Read the model definition and answer for the solid it produces. Units are mm, in the model's axes. Face numbers are marked on the shaded views. A direction names the side the tool comes from. Coordinates: 2 decimals unless noted, no trailing zeros. Loops run counter-clockwise (first coordinate to the right, second up) from the corner with the lowest first, then second, coordinate; pieces in that order, holes last. Notation, with made-up numbers: (72.5, 6.25) -> (111.5, 6.25) arc R11 cw to (111.5, 15.25) -> close; hole circle Ø6 at (-30.5, 60.25). An arc over 180 degrees is marked (long way). One line per question, with ' | ' between items. Start each with the question number.
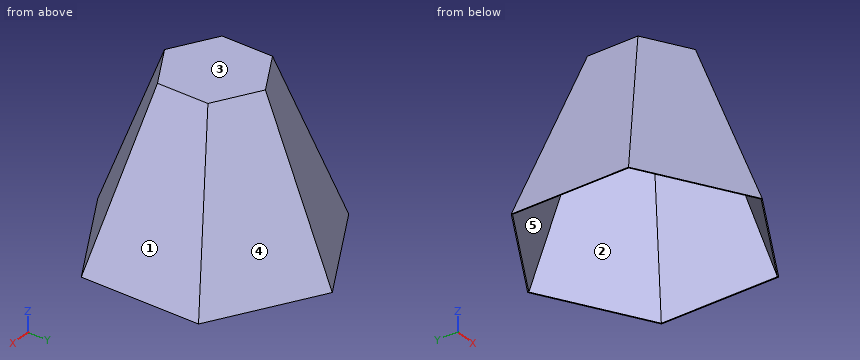
```python
from build123d import *

# Parameters (mm, degrees)
SALIENTE_EXTRUIR1_DEPTH = 125
NGULO_DE_SALIDA1_ANGLE  = 19
VACIADO1_T              = -1.4


with BuildPart() as part:
    # Croquis1 → Saliente-Extruir1 (new, symmetric)
    with BuildSketch(Plane.XY):
        Polygon((0, 75), (-64.951905284, 37.5), (-64.951905284, -37.5), (0, -75), (64.951905284, -37.5), (64.951905284, 37.5), align=None)
    extrude(amount=SALIENTE_EXTRUIR1_DEPTH, both=True)

    # Ángulo de salida1
    ngulo_de_salida1_faces = [part.faces().sort_by_distance(p)[0] for p in [
        (-32.475952642, 56.25, 0),
        (-64.951905284, 0, 0),
        (-32.475952642, -56.25, 0),
        (32.475952642, 56.25, 0),
        (64.951905284, 0, 0),
        (32.475952642, -56.25, 0),
    ]]
    draft(ngulo_de_salida1_faces, Plane.XY.offset(125), NGULO_DE_SALIDA1_ANGLE)

    # Vaciado1
    vaciado1_openings = [part.faces().sort_by_distance(p)[0] for p in [
        (0, 0, -125),
    ]]
    offset(amount=VACIADO1_T, openings=vaciado1_openings, kind=Kind.INTERSECTION)


solid = part.part
```
(1) Each of these flat-tipped pins is pushed along its axis until it touches: pin 1 Ø6 at (x, z) = (7.5, 59.5) entering from +Y; pin 2 Ø2 at (x, z) = (-62, 13) entering from +Y; pin 3 Ø5 at (y, z) = (47.5, -47) entering from +X. Where does it stop, or does it pass through?
(2) Determine the mould class of the marked faces 1, 2 and 3 for opening direction X: +X half, -X half, draft (parallel to the pull), parting line (faces both ways), or undercut.
(3) Section A-A on z = -44.5 is taken. Write down the section's boundary in (x, y), plus the area to 3 significant figures.
(4) A tool of negligible diameter and unlimited length cuts with its end or side. For the marked faces 4 and 5, from which of +Z, -Z, +X, -X, +Y, -Y can it reach the whole face along a straight path? Write none if from no direction.
(5) Section D-D on z = 84 is taken. Write down the section's boundary in (x, y).
(6) Section B-B on y = 14.5 is taken. Write down the section's boundary in (x, z).
(7) Section C-C on x = -49 is taken. Write down the section's boundary in (y, z), plus the area to 3 significant figures.
(8) Find the intervals of material crossed by probe 1 along Z at (x, y) = (-28.5, 12.5); probe 2 along X at (y, z) = (-104, -31.5); probe 3 along Y at (x, z) = (5.5, -108), in increasing order. Write a range as from..to.
Working result:
1) pin 1: stops at y = 98.82 | pin 2: stops at y = 84.44 | pin 3: stops at x = 125.04
2) face 1: +X half | face 2: undercut | face 3: draft
3) outline: (-123.32, -71.2) -> (0, -142.39) -> (123.32, -71.2) -> (123.32, 71.2) -> (0, 142.39) -> (-123.32, 71.2) -> close; hole (-121.83, -70.34) -> (0, -140.68) -> (121.83, -70.34) -> (121.83, 70.34) -> (0, 140.68) -> (-121.83, 70.34) -> close | area: 1,260 mm2
4) face 4: +Z, +X, +Y | face 5: -Z
5) outline: (-79.07, -45.65) -> (0, -91.3) -> (79.07, -45.65) -> (79.07, 45.65) -> (0, 91.3) -> (-79.07, 45.65) -> close; hole (-77.59, -44.8) -> (0, -89.59) -> (77.59, -44.8) -> (77.59, 44.8) -> (0, 89.59) -> (-77.59, 44.8) -> close
6) outline: (-151.03, -125) -> (-149.55, -125) -> (-63.95, 123.6) -> (63.95, 123.6) -> (149.55, -125) -> (151.03, -125) -> (64.95, 125) -> (-64.95, 125) -> close
7) outline: (-146.11, -125) -> (-144.4, -125) -> (-45.56, 123.6) -> (45.56, 123.6) -> (144.4, -125) -> (146.11, -125) -> (46.71, 125) -> (-46.71, 125) -> close | area: 982 mm2
8) probe 1: z = 123.6..125 | probe 2: x = -57.55..-54.58, 54.58..57.55 | probe 3: y = -164.46..-162.75, 162.75..164.46
